Part model, mm, in its own coordinate system. Face numbers are marked on the shaded views. A direction names the side the tool comes from. Round coordinates to 2 decimals unless told otherwise and drop trailing zeros. Order: outer loops, then holes, each group sorted by start corner. A loop starts at its lowest first (then second) coordinate and runs counter-clockwise, first axis right, second up. Notation, with made-up numbers: (-26.5, -39) - (23.5, -39) arc R22 ccw to (23.5, -4) - close; hole circle Ø11 at (5.5, -12.75). An arc over 180 degrees is marked (long way). Return JSON: item names as keys, results as strings. Group by question number.
Item 1: Two-plate mould, pull along X, no slides. Class the marked faces 3, 4 and 5: released by +X, released by -X, zero draft, split by the parting line, or undercut.
Item 2: Saw through at B-B on z = 28.5. List the corners of the cut face in (x, y), and give its area (3 significant figures).
Item 3: Probe probe 1 along Y at (x, z) = (27, 32); probe 2 along X at (y, z) = (-17.5, 10.5); probe 3 along Y at (x, z) = (11.5, 14.5). List the from-to ranges inside material, lowest first.
Item 4: Tool access for the marked faces 1 and 2: list every direction of +Z, -Z, +X, -X, +Y, -Y with a clear straight run to the whole face (end or side of a thin tool).
Item 5: Saw through at D-D on x = -8. List the corners of the cut face in (y, z).
Item 6: Drop flat-ended pins along their axis: pin 1 (5 mm diameter, centred on x = 21, y = -28, fed in from +Z); pin 2 (3 mm diameter, centred on x = -18, y = -9, fed in from +Z); pin 3 (3 mm diameter, centred on x = 18.5, y = 29, fed in from +Z). Give the stop position or say it passes through.
Item 7: Saw through at A-A on z = 4. State how many separate pieces and enclosed holes the cut face has, and give its area (3 significant figures).
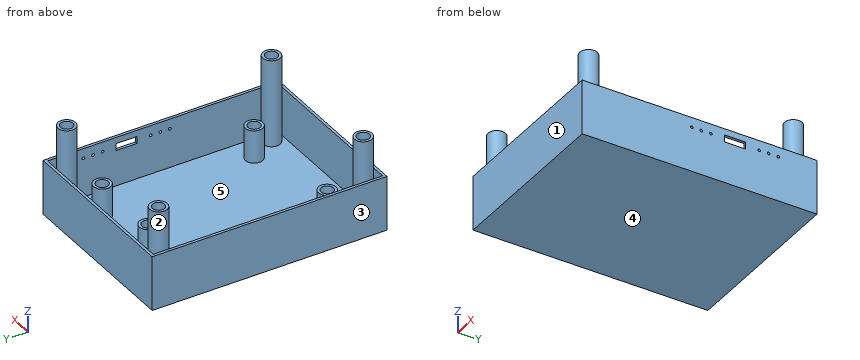
```python
from build123d import *

# Parameters (mm, degrees)
SKETCH_1_W          = 64.2
SKETCH_1_H          = 86
EXTRUDE_1_DEPTH     = 20
SKETCH_2_W          = 62.2
SKETCH_2_H          = 84
CUT_EXTRUDE_1_DEPTH = 18
SKETCH_3_R          = 3.2
EXTRUDE_2_DEPTH     = 12
SKETCH_6_R          = 2.25
CUT_EXTRUDE_4_DEPTH = 8
SKETCH_7_R          = 3.2
EXTRUDE_3_DEPTH     = 32
SKETCH_8_R          = 2.25
CUT_EXTRUDE_5_DEPTH = 8
SKETCH_11_R         = 0.5
SKETCH_11_W         = 2.6
SKETCH_11_H         = 7.6
CUT_EXTRUDE_6_DEPTH = 2


with BuildPart() as part:
    # Эскиз1 → Бобышка-Вытянуть1 (new body)
    with BuildSketch(Plane.XY):
        Rectangle(SKETCH_1_W, SKETCH_1_H)
    extrude(amount=EXTRUDE_1_DEPTH)

    # Эскиз2 → Вырез-Вытянуть1 (cut)
    with BuildSketch(Plane.XY.offset(20)):
        Rectangle(SKETCH_2_W, SKETCH_2_H)
    extrude(amount=-CUT_EXTRUDE_1_DEPTH, mode=Mode.SUBTRACT)

    # Эскиз3 → Бобышка-Вытянуть2 (add)
    with BuildSketch(Plane.XY.offset(2)):
        with Locations((-21, -28)):
            Circle(SKETCH_3_R)
        with Locations((22, -28)):
            Circle(SKETCH_3_R)
        with Locations((19, 29.5)):
            Circle(SKETCH_3_R)
        with Locations((-8, 29.5)):
            Circle(SKETCH_3_R)
    extrude(amount=EXTRUDE_2_DEPTH)

    # Эскиз6 → Вырез-Вытянуть4 (cut)
    with BuildSketch(Plane.XY.offset(14)):
        with Locations((-21, -28)):
            Circle(SKETCH_6_R)
        with Locations((-8, 29.5)):
            Circle(SKETCH_6_R)
        with Locations((19, 29.5)):
            Circle(SKETCH_6_R)
        with Locations((22, -28)):
            Circle(SKETCH_6_R)
    extrude(amount=-CUT_EXTRUDE_4_DEPTH, mode=Mode.SUBTRACT)

    # Эскиз7 → Бобышка-Вытянуть3 (add)
    with BuildSketch(Plane.XY.offset(2)):
        with Locations((-27, -37.5)):
            Circle(SKETCH_7_R)
        with Locations((27, -37.5)):
            Circle(SKETCH_7_R)
        with Locations((-27, 37.5)):
            Circle(SKETCH_7_R)
        with Locations((27, 37.5)):
            Circle(SKETCH_7_R)
    extrude(amount=EXTRUDE_3_DEPTH)

    # Эскиз8 → Вырез-Вытянуть5 (cut)
    with BuildSketch(Plane.XY.offset(34)):
        with Locations((-27, 37.5)):
            Circle(SKETCH_8_R)
        with Locations((27, 37.5)):
            Circle(SKETCH_8_R)
        with Locations((27, -37.5)):
            Circle(SKETCH_8_R)
        with Locations((-27, -37.5)):
            Circle(SKETCH_8_R)
    extrude(amount=-CUT_EXTRUDE_5_DEPTH, mode=Mode.SUBTRACT)

    # Эскиз11 → Вырез-Вытянуть6 (cut)
    with BuildSketch(Plane(origin=(32.1, 0, 0), x_dir=(0, 0, -1), z_dir=(1, 0, 0))):
        with Locations((-16.4, 21.8)):
            Circle(SKETCH_11_R)
        with Locations((-16.4, 25.3)):
            Circle(SKETCH_11_R)
        with Locations((-16.4, 28.8)):
            Circle(SKETCH_11_R)
        with Locations((-16.4, 0.65)):
            Circle(SKETCH_11_R)
        with Locations((-16.4, 4.15)):
            Circle(SKETCH_11_R)
        with Locations((-16.4, -2.85)):
            Circle(SKETCH_11_R)
        with Locations((-16.4, 13)):
            Rectangle(SKETCH_11_W, SKETCH_11_H)
    extrude(amount=-CUT_EXTRUDE_6_DEPTH, mode=Mode.SUBTRACT)


solid = part.part
```
Filled in:
{
 "1": {"face 3": "released by -X", "face 4": "zero draft", "face 5": "undercut"},
 "2": {"outline": "circle Ø6.4 at (-27, -37.5); circle Ø6.4 at (-27, 37.5); circle Ø6.4 at (27, -37.5); circle Ø6.4 at (27, 37.5); hole circle Ø4.5 at (-27, -37.5); hole circle Ø4.5 at (-27, 37.5); hole circle Ø4.5 at (27, -37.5); hole circle Ø4.5 at (27, 37.5)", "area": "65.1 mm^2"},
 "3": {"probe 1": "y = -40.7 to -39.75, -35.25 to -34.3, 34.3 to 35.25, 39.75 to 40.7", "probe 2": "x = -32.1 to -31.1, 31.1 to 32.1", "probe 3": "y = -43 to -42, 42 to 43"},
 "4": {"face 1": "+Z, -Z, +X, -X, -Y", "face 2": "+Z"},
 "5": {"outline": "(-43, 0) - (43, 0) - (43, 20) - (42, 20) - (42, 2) - (32.7, 2) - (32.7, 14) - (31.75, 14) - (31.75, 6) - (27.25, 6) - (27.25, 14) - (26.3, 14) - (26.3, 2) - (-42, 2) - (-42, 20) - (-43, 20) - close"},
 "6": {"pin 1": "stops at z = 14", "pin 2": "stops at z = 2", "pin 3": "stops at z = 6"},
 "7": {"separate pieces": "9", "enclosed holes": "1", "area": "554 mm^2"}
}
